Part model, mm, in its own coordinate system. A direction names the side the tool comes from. Coordinates: 2 decimals unless noted, no trailing zeros. Write each loop counter-clockwise with the first axis right and the second up, starting at its lowest first coordinate (ties: lowest second). Pieces come first, ordered by that corner, then holes. Notation, with made-up numbers: M 71.5,49 L 113.5,49 A26 cw 113.5,84 Z; hole C -37.5,6.5 d10. An arc over 180 degrees is marked long. Use a Markdown table: item, result. Add a question column.
Q1. Mould opens along X. For faces 6 (the flat face through (-52, -1, 1)), 7 (the flat face through (-47.2, -1, 4)), 8 (the flat face through (27, 62.2, 4)) say: released by +X, released by -X, zero draft, split by the parting line, or undercut.
Q2. Slice it at B-B on x = 39. Write the cut outline in (y, z).
Q3. Pin check, flat tips, straight feed: pin 1 Ø1.5 at (x, y) = (21, -5.5) entering from +Z; pin 2 Ø2 at (y, z) = (0, 4.5) entering from -X; pin 3 Ø3 at (x, z) = (-39, 5) entering from +Y. Stop position of each tip, or through.
Q4. Wall check: L1, parallel to Y at x = 46, z = 0.5; L2, parallel to Y at x = 32, z = 3.3; L3, parallel to X at y = -6, z = 5.2. Give the ranges that are in metal, low to high. Write a range as from..to.
Q5. Tool access for faces 1 (the flat face through (44, 53, 1)), 2 (the flat face through (49.2, -15, 4)), 3 (the flat face through (-34, 60.2, 4)), 4 (the flat face through (-19.541, 60, 2)), 5 (the flat face through (-35, 62.2, 4)): list every direction of +Z, -Z, +X, -X, +Y, -Y with a clear straight run to the whole face (end or side of a thin tool).
Q6. Slice it at D-D on x = -44.5. Write the cut outline in (y, z), then the cut area to 3 significant figures.
Q7. Slice it at A-A on z = 3.95. Write the cut outline in (x, y).
Q8. Slice it at C-C on y = -51.5. Write the cut outline in (x, z), then the cut area to 3 significant figures.
from build123d import *

# Parameters (mm, degrees)
SKETCH_1_W          = 104
SKETCH_1_H          = 130
EXTRUDE_1_DEPTH     = 3
SKETCH_2_W          = 98.4
SKETCH_2_H          = 124.4
SKETCH_2_W_2        = 94.4
SKETCH_2_H_2        = 120.4
EXTRUDE_2_DEPTH     = 2.5
SKETCH_3_W          = 16
SKETCH_3_H          = 19
SKETCH_3_W_2        = 25
SKETCH_3_H_2        = 9
CUT_EXTRUDE_1_DEPTH = 84.422119369


with BuildPart() as part:
    # 草圖1 → 填料-伸長1 (new body)
    with BuildSketch(Plane.XY):
        Rectangle(SKETCH_1_W, SKETCH_1_H)
    extrude(amount=EXTRUDE_1_DEPTH)

    # 草圖2 → 填料-伸長2 (add)
    with BuildSketch(Plane.XY.offset(3)):
        Rectangle(SKETCH_2_W, SKETCH_2_H)
        Rectangle(SKETCH_2_W_2, SKETCH_2_H_2, mode=Mode.SUBTRACT)
    extrude(amount=EXTRUDE_2_DEPTH)

    # 草圖3 → 除料-伸長1 (cut, through all)
    with BuildSketch(Plane(origin=(0, 0, 0), x_dir=(-1, 0, 0), z_dir=(0, 0, -1))):
        with Locations((-44, 43.5)):
            Rectangle(SKETCH_3_W, SKETCH_3_H)
        with Locations((7.041187405, 60.5)):
            Rectangle(SKETCH_3_W_2, SKETCH_3_H_2)
    extrude(amount=-CUT_EXTRUDE_1_DEPTH, mode=Mode.SUBTRACT)


solid = part.part
Recorded:
| question | item | result |
|---|---|---|
| 1 | face 6 | released by -X |
| 1 | face 7 | undercut |
| 1 | face 8 | zero draft |
| 2 | outline | M -65,0 L 34,0 L 34,3 L -60.2,3 L -60.2,5.5 L -62.2,5.5 L -62.2,3 L -65,3 Z; M 53,0 L 65,0 L 65,3 L 62.2,3 L 62.2,5.5 L 60.2,5.5 L 60.2,3 L 53,3 Z |
| 3 | pin 1 | z = 3 |
| 3 | pin 2 | x = -49.2 |
| 3 | pin 3 | y = 62.2 |
| 4 | L1 | -65..34, 53..65 |
| 4 | L2 | -62.2..-60.2, 60.2..62.2 |
| 4 | L3 | -49.2..-47.2, 47.2..49.2 |
| 5 | face 1 | +Z, -Z, +X |
| 5 | face 2 | +Z, +X, +Y, -Y |
| 5 | face 3 | +Z |
| 5 | face 4 | +Z, -Z, +Y |
| 5 | face 5 | +Z, +X, -X, +Y |
| 6 | outline | M -65,0 L 65,0 L 65,3 L 62.2,3 L 62.2,5.5 L 60.2,5.5 L 60.2,3 L -60.2,3 L -60.2,5.5 L -62.2,5.5 L -62.2,3 L -65,3 Z |
| 6 | area | 400 mm² |
| 7 | outline | M -49.2,-62.2 L 49.2,-62.2 L 49.2,34 L 47.2,34 L 47.2,-60.2 L -47.2,-60.2 L -47.2,60.2 L -19.54,60.2 L -19.54,62.2 L -49.2,62.2 Z; M 5.46,60.2 L 47.2,60.2 L 47.2,53 L 49.2,53 L 49.2,62.2 L 5.46,62.2 Z |
| 8 | outline | M -52,0 L 52,0 L 52,3 L 49.2,3 L 49.2,5.5 L 47.2,5.5 L 47.2,3 L -47.2,3 L -47.2,5.5 L -49.2,5.5 L -49.2,3 L -52,3 Z |
| 8 | area | 322 mm² |
